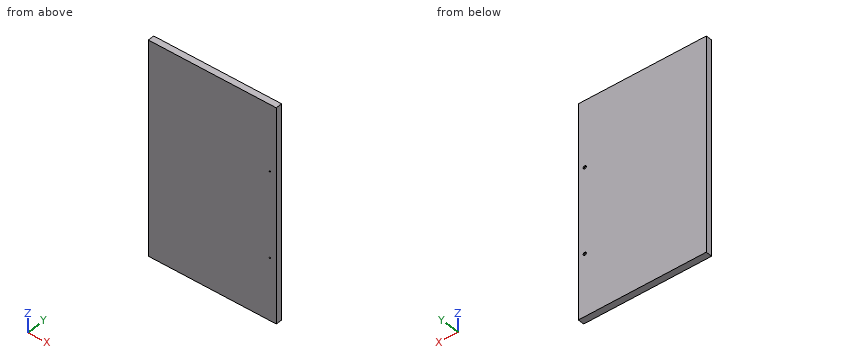
Autodesk Inventor part; units mm, degrees
ref_plane "YZ Plane" through (0, 0, 0) normal (1, 0, 0) x (0, 1, 0)
ref_plane "XZ Plane" through (0, 0, 0) normal (0, 1, 0) x (-1, 0, 0)
ref_plane "XY Plane" through (0, 0, 0) normal (0, 0, 1) x (1, 0, 0)
sketch "草圖1" plane through (0, 0, 0) normal (0, 1, 0) x (-1, 0, 0)
  line L0 (0, 0) -> (600, 0)
  line L1 (600, 0) -> (600, -1000)
  line L2 (600, -1000) -> (0, -1000)
  line L3 (0, -1000) -> (0, 0)
  line L4 (0, 0) -> (30, 0)
  line L5 (0, -310) -> (0, 0)
  line L6 (0, -710) -> (0, -310)
  circle A0 centre (30, -310) radius 7.5
  circle A1 centre (30, -710) radius 7.5
  line L7 (0, 0) -> (15, 0)
  line L8 (15, 0) -> (15, -15)
  line L9 (15, -15) -> (0, -15)
  line L10 (0, -15) -> (0, 0)
  line L11 (15, -15) -> (585, -15)
  line L12 (585, -15) -> (585, -985)
  line L13 (585, -985) -> (15, -985)
  line L14 (15, -985) -> (15, -15)
  circle A2 centre (30, -710) radius 3
  circle A3 centre (30, -310) radius 3
  dimension "d0" = 1000
  dimension "d1" = 600
  dimension "d6" = 15
  dimension "d7" = 15
  dimension "d8" = 310
  dimension "d9" = 30
  dimension "d10" = 400
  dimension "d11" = 30
  dimension "d14" = 15
  dimension "d15" = 15
  dimension "d16" = 570
  dimension "d17" = 970
  dimension "d26" = 6
  dimension "d27" = 6
extrude "擠出1" add sketch "草圖1" against normal blind 30 contours L0 L8 L9 L3 | L11 L12 L13 L14 | L0 L1 L2 L3 L9 L8
extrude "擠出2" add sketch "草圖1" against normal blind 30 contours A0 | A1 | A2 | A3
extrude "擠出3" cut sketch "草圖1" against normal blind 25 contours L11 L12 L13 L14
extrude "擠出4" add sketch "草圖1" against normal blind 5 contours L0 L8 L9 L3 | L11 L12 L13 L14 | L0 L1 L2 L3 L9 L8 | A0 | A1 | A2 | A3
extrude "擠出5" cut sketch "草圖1" against normal blind 25 contours A0 | A1 | A2 | A3
extrude "擠出6" cut sketch "草圖1" against normal through all contours A2 | A3
properties part number "Body Actuator"
Design review of the part built by this model. Coordinates are the model's own, in mm. Coordinates: 2 decimals unless noted, no trailing zeros. Order: outer loops, then holes, each group sorted by start corner. A loop starts at its lowest first (then second) coordinate and runs counter-clockwise, first axis right, second up. Notation, with made-up numbers: (64.25, 9) -> (119.25, 9) arc R31 ccw to (119.25, 33) -> close; hole circle Ø11 at (28.25, 9). An arc over 180 degrees is marked (long way). Use one line per item in the form item = value. Start each with the question number.
(1) Add section A-A on z = -657. State the section outline as (x, y) points, plus the area to 3 significant figures.
(2) Insertion check: pin 1 (5.5 mm diameter, centred on x = -30, z = -310, fed in from -Y); pin 2 (9.5 mm diameter, centred on x = -30, z = -710, fed in from +Y). Each pin has a flat end and moves straight along its axis. Give the tip position at first contact, or say it passes through.
(3) Add section B-B on y = -16. State the section outline as (x, z) points, plus the area to 3 significant figures.
(4) For probe 1 along Z at (x, y) = (-30, -26.6); probe 2 along Z at (x, y) = (-30, -2.3); probe 3 along X at (y, z) = (-2.05, -310), list the stretches that pass through material, from the lowest coordinate up.
Answer block:
q1.outline = (-600, -30) -> (0, -30) -> (0, 0) -> (-600, 0) -> close; hole (-585, -25) -> (-15, -25) -> (-15, -5) -> (-585, -5) -> close
q1.area = 6,600 mm²
q2.pin_1 = through
q2.pin_2 = -25
q3.outline = (-600, -1000) -> (0, -1000) -> (0, 0) -> (-600, 0) -> close; hole (-585, -985) -> (-15, -985) -> (-15, -15) -> (-585, -15) -> close
q3.area = 47,100 mm²
q4.probe_1 = -1000 to -713, -707 to -313, -307 to 0
q4.probe_2 = -1000 to -717.5, -702.5 to -317.5, -302.5 to 0
q4.probe_3 = -600 to -37.5, -22.5 to 0
